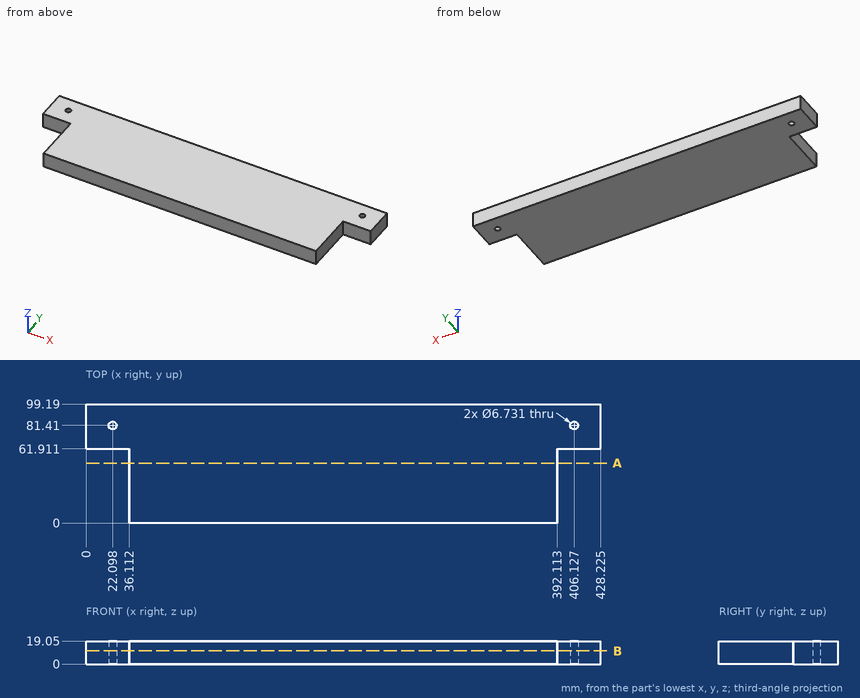
Verification items for this drawing (mm, ordinates from the low corner). Coordinates: 2 decimals unless noted, no trailing zeros. Write each loop counter-clockwise with the first axis right and the second up, starting at its lowest first coordinate (ties: lowest second). Pieces come first, ordered by that corner, then holes. Notation, with made-up numbers: M -10.5,51.5 L 31.5,51.5 A9 ccw 31.5,56.5 Z; hole C -4.75,57.25 d7. An arc over 180 degrees is marked long. Use one line per item in the form item = value. Start each with the question number.
1) Section check B-B on z = 11. Enter the section's corners in (x, y) (1 decimal), and give its area (3 significant figures).
2) Thickness scan on probe 1 along X at (y, z) = (23, 7); probe 2 along X at (y, z) = (82.5, 3.25) (1 decimal). Record the ranges inside material, lowest first. Write a range as from..to.
3) Go/stop test with flat-tipped pins: pin 1 Ø6 at (x, y) = (22.1, 81.41) entering from +Z; pin 2 Ø5.5 at (x, z) = (11.5, 8) entering from -Y; pin 3 Ø1 at (y, z) = (13.5, 12.5) entering from -X; pin 4 Ø9.5 at (y, z) = (32, 7.5) entering from +X. Record where each tip stops, or that it passes through.
4) Section check A-A on y = 50. Enter the section's corners in (x, z).
Responses:
q1.outline = M 0,61.9 L 36.1,61.9 L 36.1,0 L 392.1,0 L 392.1,61.9 L 428.2,61.9 L 428.2,99.2 L 0,99.2 Z; hole C 22.1,81.4 d6.7; hole C 406.1,81.4 d6.7
q1.area = 37,900 mm2
q2.probe_1 = 36.11..392.11
q2.probe_2 = 0..18.9, 25.3..402.9, 409.3..428.2
q3.pin_1 = through
q3.pin_2 = 61.91
q3.pin_3 = 36.11
q3.pin_4 = 392.11
q4.outline = M 36.11,0 L 392.11,0 L 392.11,19.05 L 36.11,19.05 Z
